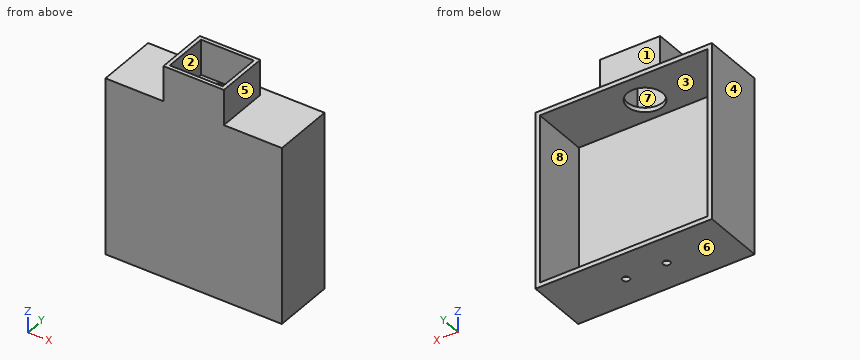
```python
from build123d import *

# Parameters (mm, degrees)
SKETCH_1_W               = 100
SKETCH_1_H               = 100
EXTRUDE_1_DEPTH          = 35
SKETCH_2_W               = 95
SKETCH_2_H               = 95
CUT_EXTRUDE_1_DEPTH      = 32
CUT_EXTRUDE_2_DEPTH      = 118.153745139
CUT_EXTRUDE_2_DEPTH_BACK = 32
SKETCH_3_R               = 10
SKETCH_4_R               = 2
CUT_EXTRUDE_3_DEPTH      = 32
EXTRUDE_2_DEPTH          = 20
SKETCH_6_W               = 29.993378998
SKETCH_6_H               = 25.557725667
CUT_EXTRUDE_4_DEPTH      = 118.153745139


with BuildPart() as part:
    # Эскиз1 → Бобышка-Вытянуть1 (new body)
    with BuildSketch(Plane(origin=(0, 0, 0), x_dir=(1, 0, 0), z_dir=(0, 1, 0))):
        Rectangle(SKETCH_1_W, SKETCH_1_H)
    extrude(amount=EXTRUDE_1_DEPTH)

    # Эскиз2 → Вырез-Вытянуть1 (cut)
    with BuildSketch(Plane(origin=(0, 35, 0), x_dir=(1, 0, 0), z_dir=(0, 1, 0))):
        Rectangle(SKETCH_2_W, SKETCH_2_H)
    extrude(amount=-CUT_EXTRUDE_1_DEPTH, mode=Mode.SUBTRACT)

    # Эскиз3 → Вырез-Вытянуть2 (cut, two sides: drawn at the far end of the back side and taken through both)
    with BuildSketch(Plane.XY.offset(50).offset(-CUT_EXTRUDE_2_DEPTH_BACK)):
        with Locations(Location((0, 17.5, 0), (0, 0, 180))):
            Circle(SKETCH_3_R)
    extrude(amount=CUT_EXTRUDE_2_DEPTH + CUT_EXTRUDE_2_DEPTH_BACK, mode=Mode.SUBTRACT)

    # Эскиз4 → Вырез-Вытянуть3 (cut)
    with BuildSketch(Plane(origin=(0, 0, -50), x_dir=(-1, 0, 0), z_dir=(0, 0, -1))):
        with Locations((-10.76282056, 17.5)):
            Circle(SKETCH_4_R)
        with Locations((12.23717944, 17.5)):
            Circle(SKETCH_4_R)
    extrude(amount=-CUT_EXTRUDE_3_DEPTH, mode=Mode.SUBTRACT)

    # Эскиз5 → Бобышка-Вытянуть2 (add)
    with BuildSketch(Plane.XY.offset(50)):
        Polygon((-17.118009843, 5.199633646), (-17.118009843, 0), (17.118009843, 0), (17.118009843, 5.199633646), (17.118009843, 29.800366354), (-17.118009843, 29.800366354), align=None)
    extrude(amount=EXTRUDE_2_DEPTH)

    # Эскиз6 → Вырез-Вытянуть4 (cut, through all)
    with BuildSketch(Plane(origin=(0, 0, 50), x_dir=(-1, 0, 0), z_dir=(0, 0, -1))):
        with Locations((0, 14.900183178)):
            Rectangle(SKETCH_6_W, SKETCH_6_H)
    extrude(amount=-CUT_EXTRUDE_4_DEPTH, mode=Mode.SUBTRACT)


solid = part.part
```
Could you check a few things on this model? Use its own coordinates, in mm. Face numbers are marked on the shaded views. A direction names the side the tool comes from. Round coordinates to 2 decimals unless told otherwise and drop trailing zeros. Loops run counter-clockwise (first coordinate to the right, second up) from the corner with the lowest first, then second, coordinate; pieces in that order, holes last. Notation, with made-up numbers: M 57.5,32 L 95.5,32 A23 cw 95.5,62 Z; hole C 14,70 d11. An arc over 180 degrees is marked long. Put each result on its own line as item: value.
Q1. I need wall thicknesses on probe 1 along Z at (x, y) = (-13, 11); probe 2 along Y at (x, z) = (-14, 64). Which ranges of each line are inside material? Lowest first, please.
Check result:
probe 1: -50 to -47.5, 47.5 to 50
probe 2: 0 to 2.12, 27.68 to 29.8
Q2. Imagine slicing it at A-A (x = -6). Write out the boundary of the cut face in (y, z), then the cut area to 3 significant figures.
Check result:
outline: M 0,-50 L 35,-50 L 35,-47.5 L 3,-47.5 L 3,47.5 L 9.5,47.5 L 9.5,50 L 2.12,50 L 2.12,70 L 0,70 Z; M 25.5,47.5 L 35,47.5 L 35,50 L 29.8,50 L 29.8,70 L 27.68,70 L 27.68,50 L 25.5,50 Z
area: 505 mm2
Q3. Imagine slicing it at C-C (y = 6). Write out the boundary of the cut face in (x, z).
Check result:
outline: M -50,-50 L 50,-50 L 50,50 L 17.12,50 L 17.12,70 L 15,70 L 15,50 L -15,50 L -15,70 L -17.12,70 L -17.12,50 L -50,50 Z; hole M -47.5,-47.5 L 47.5,-47.5 L 47.5,47.5 L -47.5,47.5 Z
Q4. For pin 1 (22 mm diameter, centred on x = 2, z = 64.5, fed in from +Y); pin 2 (8 mm diameter, centred on x = 6.5, z = 24.5, fed in from +Y); pin 3 (16 mm diameter, centred on y = 19.5, z = 60.5, fed in from -X); pin 4 (22 mm diameter, centred on x = -7.5, z = 60, fed in from -Y), each with a flat end and sliding along its axis, tell me the tip position at first contact or that it passes through.
Check result:
pin 1: y = 29.8
pin 2: y = 3
pin 3: x = -17.12
pin 4: y = 0
Q5. Imagine slicing it at B-B (y = 17.5). Write out the boundary of the cut face in (x, z).
Check result:
outline: M -50,-50 L -14.24,-50 L -14.24,-47.5 L -47.5,-47.5 L -47.5,47.5 L -10,47.5 L -10,50 L -15,50 L -15,70 L -17.12,70 L -17.12,50 L -50,50 Z; M -10.24,-50 L 8.76,-50 L 8.76,-47.5 L -10.24,-47.5 Z; M 10,47.5 L 47.5,47.5 L 47.5,-47.5 L 12.76,-47.5 L 12.76,-50 L 50,-50 L 50,50 L 17.12,50 L 17.12,70 L 15,70 L 15,50 L 10,50 Z
Q6. Thinking about a two-plate mould opening in Z: for the marked faces 6, 7 and 8, which applies, released by +Z, released by -Z, zero draft, split by the parting line, or undercut?
Check result:
face 6: released by -Z
face 7: zero draft
face 8: undercut
Q7. On a 3-axis mill with a long thin cutter (end or side, diameter ignored), from which of +Z, -Z, +X, -X, +Y, -Y can I reach the whole of each face in a straight line? I mean the marked faces 1, 2, 3, 4 and 5. Say none if no direction works.
Check result:
face 1: +Z, +X, -X, +Y
face 2: +Z
face 3: +Y
face 4: +Z, -Z, -X, +Y, -Y
face 5: +Z, +X, +Y, -Y
Q8. Imagine slicing it at D-D (z = -6.5). Write out the boundary of the cut face in (x, y), then the cut area to 3 significant figures.
Check result:
outline: M -50,0 L 50,0 L 50,35 L 47.5,35 L 47.5,3 L -47.5,3 L -47.5,35 L -50,35 Z
area: 460 mm2
